Source: CAD feature listing. Evaluate the final solid. Frame: model axes, mm. Face numbers are marked on the shaded views. Round coordinates to 2 decimals unless told otherwise and drop trailing zeros. Loops run counter-clockwise (first coordinate to the right, second up) from the corner with the lowest first, then second, coordinate; pieces in that order, holes last.
(1) Material intervals for probe 1 along Y at (x, z) = (0, -4.25) (3 decimals); probe 2 along Y at (x, z) = (17, -8.25); probe 3 along X at (y, z) = (-23, -6), sorted ascending.
(2) Mould query, pull axis Y, two halves, no side actions, for the marked faces 1 and 2. Classes: pulls with the +Y half, pulls with the -Y half, needs draft (parallel to the pull), parting line crosses it, or undercut.
(3) Section A-A, the plane z = -3.75. Return the cut outline in (x, y) (3 decimals), plus the area to 3 significant figures.
(4) First-contact query: pin 1 Ø8 at (y, z) = (-19, 5) entering from +X; pin 2 Ø8 at (x, z) = (-5.5, 7) entering from +Y; pin 3 Ø2 at (y, z) = (-4.5, -7.5) entering from -X. Flat tips, straight axial feed; report the tip coordinate or a pass-through.
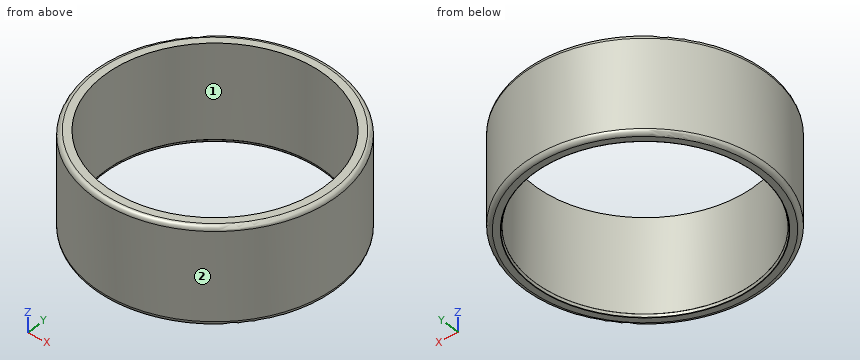
```python
from build123d import *

# Parameters (mm, degrees)
FILLET1_R = 0.1


with BuildPart() as part:
    # Sketch1 → Revolve1 (revolve)
    with BuildSketch(Plane(origin=(0, 0, 0), x_dir=(0, 0, -1), z_dir=(1, 0, 0)), mode=Mode.PRIVATE) as revolve1_sk:
        with BuildLine():
            Line((10, 27.825), (-10, 27.825))
            ThreePointArc((-10, 27.825), (-10.707106781, 27.532106781), (-11, 26.825))
            Line((-11, 26.825), (-11, 25.125))
            Line((-11, 25.125), (10.368080194, 25.125))
            Line((10.368080194, 25.125), (11, 25.355))
            Line((11, 25.355), (11, 26.825))
            ThreePointArc((11, 26.825), (10.707106781, 27.532106781), (10, 27.825))
        make_face()
    revolve(revolve1_sk.sketch.rotate(Axis((0, 0, 55), (0, 0, -1)), 90), axis=Axis((0, 0, 55), (0, 0, -1)))

    # Fillet1
    fillet1_edges = [part.edges().sort_by_distance(p)[0] for p in [
        (-25.355, 0, -11),
        (-25.125, 0, -10.368080194),
    ]]
    fillet(fillet1_edges, radius=FILLET1_R)


solid = part.part
```
Output values:
1. probe 1: y = -27.825 to -25.125, 25.125 to 27.825
1. probe 2: y = -22.03 to -18.5, 18.5 to 22.03
1. probe 3: x = -15.66 to -10.11, 10.11 to 15.66
2. face 1: undercut
2. face 2: parting line crosses it
3. outline: circle Ø55.65 at (0, 0); hole circle Ø50.25 at (0, 0)
3. area: 449 mm2
4. pin 1: stops at x = 23.44
4. pin 2: stops at y = 27.78
4. pin 3: stops at x = -27.6
